```python
from build123d import *

# Parameters (mm, degrees)
SKETCH1_R           = 31
BOSS_EXTRUDE1_DEPTH = 10
BOSS_EXTRUDE3_DEPTH = 10
CUT_EXTRUDE2_DEPTH  = 20
SKETCH8_R           = 40
BOSS_EXTRUDE4_DEPTH = 10
SKETCH9_W           = 7.5
SKETCH9_H           = 5
BOSS_EXTRUDE5_DEPTH = 10
CUT_EXTRUDE3_DEPTH  = 10


with BuildPart() as part:
    # Sketch1 → Boss-Extrude1 (new body)
    with BuildSketch(Plane(origin=(0, 0, 0), x_dir=(1, 0, 0), z_dir=(0, 1, 0))):
        with Locations(Location((0, 0, 0), (0, 0, 270))):
            Circle(SKETCH1_R)
    extrude(amount=BOSS_EXTRUDE1_DEPTH)

    # Sketch6 → Boss-Extrude3 (add)
    with BuildSketch(Plane(origin=(0, 0, 0), x_dir=(-1, 0, 0), z_dir=(0, -1, 0))):
        Polygon((15, 0), (15, -10), (-15, -10), (-15, 0), (-15, 10), (15, 10), align=None)
    extrude(amount=BOSS_EXTRUDE3_DEPTH)

    # Sketch7 → Cut-Extrude2 (cut)
    with BuildSketch(Plane(origin=(0, 0, -10), x_dir=(-1, 0, 0), z_dir=(0, 0, -1))):
        Polygon((10, -5), (5, -5), (5, 0), (15, 0), (15, -10), align=None)
        Polygon((-5, 0), (-15, 0), (-15, -10), (-10, -5), (-5, -5), align=None)
    extrude(amount=-CUT_EXTRUDE2_DEPTH, mode=Mode.SUBTRACT)

    # Sketch8 → Boss-Extrude4 (add)
    with BuildSketch(Plane.XZ):
        with Locations(Location((0, 0, 0), (0, 0, 270))):
            Circle(SKETCH8_R)
        Polygon((15, -10), (22.5, -10), (22.5, 10), (15, 10), (-15, 10), (-22.5, 10), (-22.5, -10), (-15, -10), align=None, mode=Mode.SUBTRACT)
    extrude(amount=BOSS_EXTRUDE4_DEPTH)

    # Sketch9 → Boss-Extrude5 (add)
    with BuildSketch(Plane.XZ.offset(10)):
        with Locations((-18.75, 7.5)):
            Rectangle(SKETCH9_W, SKETCH9_H)
        with Locations((18.75, 7.5)):
            Rectangle(SKETCH9_W, SKETCH9_H)
        with Locations((18.75, -7.5)):
            Rectangle(SKETCH9_W, SKETCH9_H)
        with Locations((-18.75, -7.5)):
            Rectangle(SKETCH9_W, SKETCH9_H)
        Polygon((-15, 5), (0, 5), (15, 5), (15, 10), (-15, 10), align=None)
        Polygon((15, -10), (15, -5), (0, -5), (-15, -5), (-15, -10), align=None)
    extrude(amount=-BOSS_EXTRUDE5_DEPTH)

    # Sketch10 → Cut-Extrude3 (cut)
    with BuildSketch(Plane.XZ.offset(10)):
        Polygon((-22.5, -5), (-39.686269666, -5), (-48.180542602, -5), (-48.180542602, 5), (-22.5, 5), align=None)
        Polygon((22.5, 5), (48.180542602, 5), (48.180542602, -5), (39.686269666, -5), (22.5, -5), align=None)
    extrude(amount=-CUT_EXTRUDE3_DEPTH, mode=Mode.SUBTRACT)


solid = part.part
```
Here's how the part is built. I have some questions about the finished solid (model axes, mm). A direction names the side the tool comes from. Give positions to 0.01 mm unless a question says otherwise; leave off trailing zeros. Loops run counter-clockwise (first coordinate to the right, second up) from the corner with the lowest first, then second, coordinate; pieces in that order, holes last. Notation, with made-up numbers: M 29.5,-6.75 L 43.5,-6.75 A27 cw 43.5,17.25 Z; hole C 49,71 d1. An arc over 180 degrees is marked long. Return JSON: item names as keys, results as strings.
Item 1: On a 3-axis mill with a long thin cutter (end or side, diameter ignored), from which of +Z, -Z, +X, -X, +Y, -Y can I reach the whole of each face in a straight line? I mean faces 1 (the flat face through (0.2, 0, -31.5)), 2 (the flat face through (-8, -5, 0)), 3 (the flat face through (5, -3, 0)), 4 (the cylindrical face through (30.736, 4.93, -4.036)). Say none if no direction works.
A:
{"face 1": "-Z, +Y", "face 2": "-X", "face 3": "+X", "face 4": "+Y"}
Item 2: Imagine slicing it at C-C on x = 0. List the corners of the cut face in (y, z) for me, then the cut area to 3 significant figures.
A:
{"outline": "M -10,-40 L 0,-40 L 0,-31 L 10,-31 L 10,31 L 0,31 L 0,40 L -10,40 Z", "area": "1,420 mm^2"}
Item 3: Imagine slicing it at B-B on z = 0. List the corners of the cut face in (x, y) for me, then the cut area to 3 significant figures.
A:
{"outline": "M -31,0 L -5,0 L -5,-5 L -10,-5 L -15,-10 L 15,-10 L 10,-5 L 5,-5 L 5,0 L 31,0 L 31,10 L -31,10 Z", "area": "795 mm^2"}
Item 4: Thinking about a two-plate mould opening in Z: for faces 5 (the flat face through (-23, -5, 5)), 6 (the cylindrical face through (-0.81, -4.93, -39.99)), 7 (the flat face through (0, 0, 32)), 8 (the flat face through (-13, -8, 0)), which applies, released by +Z, released by -Z, zero draft, split by the parting line, or undercut?
A:
{"face 5": "undercut", "face 6": "released by -Z", "face 7": "zero draft", "face 8": "undercut"}
Item 5: I'm going to push flat-ended pins straight in: pin 1 Ø5 at (x, y) = (-30, -6.5) entering from -Z; pin 2 Ø4 at (y, z) = (-2.5, 26.5) entering from +X; pin 3 Ø12 at (y, z) = (-2.5, -6) entering from +X; pin 4 Ø2.5 at (y, z) = (-2, 1.5) entering from +X. Where does each tip first touch, or does it pass through?
A:
{"pin 1": "stops at z = -29.05", "pin 2": "stops at x = 31.62", "pin 3": "stops at x = 39.69", "pin 4": "stops at x = 5"}
Item 6: Imagine slicing it at D-D on y = 5.75. List the corners of the cut face in (x, z) for me.
A:
{"outline": "C 0,0 d62"}
Item 7: Please list where these lines run through material, in increasing order: line 1 (Y direction, x = -28, z = 26); line 2 (Y direction, x = -18, z = -2); line 3 (Z direction, x = -10, y = -1).
A:
{"line 1": "y = -10 to 0", "line 2": "y = 0 to 10", "line 3": "z = -38.73 to -5, 5 to 38.73"}
Item 8: Imagine slicing it at A-A on y = -7. List the corners of the cut face in (x, z) for me, then the cut area to 3 significant figures.
A:
{"outline": "M -39.69,-5 A40 ccw 39.69,-5 L 12,-5 L 12,5 L 39.69,5 A40 ccw -39.69,5 L -12,5 L -12,-5 Z", "area": "4,470 mm^2"}
